Part model, mm, in its own coordinate system. Coordinates: 2 decimals unless noted, no trailing zeros. Loops run counter-clockwise (first coordinate to the right, second up) from the corner with the lowest first, then second, coordinate; pieces in that order, holes last. Notation, with made-up numbers: (62.5, 70.25) -> (114.5, 70.25) arc R10 ccw to (114.5, 78.25) -> close; hole circle Ø1 at (64, 73.5). An arc over 180 degrees is marked (long way). One line per item, written item: value. Start each with the question number.
Autodesk Inventor part; units mm, degrees
ref_plane "YZ Plane" through (0, 0, 0) normal (1, 0, 0) x (0, 1, 0)
ref_plane "XZ Plane" through (0, 0, 0) normal (0, 1, 0) x (-1, 0, 0)
ref_plane "XY Plane" through (0, 0, 0) normal (0, 0, 1) x (1, 0, 0)
sketch "Sketch1" plane through (0, 0, 0) normal (0, 1, 0) x (-1, 0, 0)
  line L0 (83.5, 19.65) -> (-85, 19.65)
  line L1 (-85, 19.65) -> (-85, -19.65)
  line L2 (-85, -19.65) -> (83.5, -19.65)
  line L3 (83.5, -19.65) -> (83.5, 19.65)
  line L4 (19.05, 0) -> (-17.4625, 0) construction
  line L5 (-0.75, 11.1125) -> (-0.75, -12.7) construction
  circle A0 centre (-82.75, 17.4) radius 1.5
  circle A1 centre (-82.75, -17.4) radius 1.5
  circle A2 centre (81.25, 17.4) radius 1.5
  circle A3 centre (81.25, -17.4) radius 1.5
  circle A4 centre (46.95, 17.4) radius 1.5
  circle A5 centre (46.95, -17.4) radius 1.5
  circle A6 centre (-48.45, -17.4) radius 1.5
  circle A7 centre (-48.45, 15.9) radius 1.5
  point P0 (0, 0)
  dimension "d0" = 168.5
  dimension "d1" = 39.3
  dimension "d2" = 3
  dimension "d3" = 2.25
  dimension "d4" = 2.25
  dimension "d7" = 2.25
  dimension "d16" = 3
  dimension "d17" = 34.3
  dimension "d18" = 3
  dimension "d19" = 3
  dimension "d20" = 34.3
  dimension "d21" = 3
extrude "Extrusion1" add sketch "Sketch1" along normal blind 2 contours L3 L2 L1 L0 | A2 | A3 | A4 | A5 | A6 | A7
extrude "Extrusion2" cut sketch "Sketch1" along normal blind 2 contours A2 | A3
sketch "Sketch2" plane through (0, 2, 0) normal (0, 1, 0) x (1, 0, 0)
  line L0 (-93.5, -10) -> (-73.5, -10)
  line L1 (-73.5, -10) -> (-73.5, 10)
  line L2 (-73.5, 10) -> (-93.5, 10)
  line L3 (-93.5, 10) -> (-93.5, -10)
  line L4 (-83.5, 19.65) -> (-83.5, -19.65)
  line L5 (-93.5, -10) -> (-73.5, 10) construction
  line L6 (-73.5, -10) -> (-93.5, 10) construction
  line L7 (75, -10) -> (95, -10)
  line L8 (95, -10) -> (95, 10)
  line L9 (95, 10) -> (75, 10)
  line L10 (75, 10) -> (75, -10)
  line L11 (85, -19.65) -> (85, 19.65)
  line L12 (75, -10) -> (95, 10) construction
  line L13 (95, -10) -> (75, 10) construction
  point P0 (0, 0)
  point P1 (-83.5, 0)
  point P2 (85, 0)
  point P3 (-83.5, 10)
  point P4 (-83.5, -10)
  point P5 (85, -10)
  point P6 (85, 10)
  dimension "d10" = 20
  dimension "d11" = 20
  dimension "d12" = 20
  dimension "d13" = 20
extrude "Extrusion3" cut sketch "Sketch2" against normal blind 2 contours L4 L2 L1 L0 | L10 L9 L11 L7
sketch "Sketch3" plane through (0, 2, 0) normal (0, 1, 0) x (1, 0, 0)
  point P0 (0, 0)
extrude "Extrusion4" cut sketch "Sketch1" along normal blind 2 contours A4 | A5 | A6 | A7
properties part number "Casis Tengah_3DPrint"
1) Pin check, flat tips, straight feed: pin 1 Ø1 at (y, z) = (1, 4) entering from -X; pin 2 Ø1 at (y, z) = (0.5, -3) entering from +X. Stop position of each tip, or through.
2) Probe line 1 (Z direction, x = 48.45, y = 0.8); line 2 (Z direction, x = -46.95, y = 1.25); line 3 (Z direction, x = -81.25, y = 1.5). List the from-to ranges inside material, lowest first. Write a range as from..to.
3) Slice it at B-B (x = 48.45). Give the cut face in (y, z).
4) Slice it at D-D (x = 82.75). Give the cut face in (y, z).
5) Slice it at A-A (z = -17.4). Give the cut face in (x, y).
6) Pull direction X, two halves, no side cores. Call faces 1 (the flat face through (2, 0, 0)), 2 (the cylindrical face through (-82.68, 0.99, 16.95)), 3 (the cylindrical face through (47.02, 0.99, 15.45)): +X half, -X half, draft (parallel to the pull), parting line (faces both ways), or undercut.
7) Slice it at C-C (y = 0.55). State how many separate pieces and enclosed holes the cut face has, then the cut area to 3 significant figures.
Check sheet entries:
1. pin 1: stops at x = -73.5
1. pin 2: stops at x = 75
2. line 1: z = -19.65..-18.9, -15.9..14.4, 17.4..19.65
2. line 2: z = -19.65..-18.9, -15.9..15.9, 18.9..19.65
2. line 3: z = -19.65..-18.9, -15.9..-10, 10..15.9, 18.9..19.65
3. outline: (0, -19.65) -> (2, -19.65) -> (2, -18.9) -> (0, -18.9) -> close; (0, -15.9) -> (2, -15.9) -> (2, 14.4) -> (0, 14.4) -> close; (0, 17.4) -> (2, 17.4) -> (2, 19.65) -> (0, 19.65) -> close
4. outline: (0, -19.65) -> (2, -19.65) -> (2, -18.9) -> (0, -18.9) -> close; (0, -15.9) -> (2, -15.9) -> (2, -10) -> (0, -10) -> close; (0, 10) -> (2, 10) -> (2, 15.9) -> (0, 15.9) -> close; (0, 18.9) -> (2, 18.9) -> (2, 19.65) -> (0, 19.65) -> close
5. outline: (-83.5, 0) -> (-82.75, 0) -> (-82.75, 2) -> (-83.5, 2) -> close; (-79.75, 0) -> (-48.45, 0) -> (-48.45, 2) -> (-79.75, 2) -> close; (-45.45, 0) -> (46.95, 0) -> (46.95, 2) -> (-45.45, 2) -> close; (49.95, 0) -> (81.25, 0) -> (81.25, 2) -> (49.95, 2) -> close; (84.25, 0) -> (85, 0) -> (85, 2) -> (84.25, 2) -> close
6. face 1: draft
6. face 2: undercut
6. face 3: undercut
7. separate pieces: 1
7. enclosed holes: 8
7. area: 6,170 mm^2
